```python
from build123d import *

# Parameters (mm, degrees)
SKETCH1_W           = 236
SKETCH1_H           = 236
BOSS_EXTRUDE1_DEPTH = 240
SHELL1_T            = -40
FILLET1_R           = 23
FILLET2_R           = 30
SKETCH3_W           = 80
SKETCH3_H           = 120
CUT_EXTRUDE2_DEPTH  = 240


with BuildPart() as part:
    # Sketch1 → Boss-Extrude1 (new body)
    with BuildSketch(Plane(origin=(0, 0, 0), x_dir=(1, 0, 0), z_dir=(0, 1, 0))):
        with Locations((2.531496063, -48.329724409)):
            Rectangle(SKETCH1_W, SKETCH1_H)
    extrude(amount=BOSS_EXTRUDE1_DEPTH)

    # Shell1
    shell1_openings = [part.faces().sort_by_distance(p)[0] for p in [
        (2.531496063, 240, 48.329724409),
    ]]
    offset(amount=SHELL1_T, openings=shell1_openings, kind=Kind.INTERSECTION)

    # Fillet1
    fillet1_edges = [part.edges().sort_by_distance(p)[0] for p in [
        (-75.468503937, 40, 48.329724409),
        (-75.468503937, 140, -29.670275591),
        (2.531496063, 40, 126.329724409),
        (-75.468503937, 140, 126.329724409),
        (80.531496063, 40, 48.329724409),
        (80.531496063, 140, 126.329724409),
        (2.531496063, 40, -29.670275591),
        (80.531496063, 140, -29.670275591),
    ]]
    fillet(fillet1_edges, radius=FILLET1_R)

    # Fillet2
    fillet2_edges = [part.edges().sort_by_distance(p)[0] for p in [
        (2.531496063, 0, -69.670275591),
        (120.531496063, 0, 48.329724409),
        (2.531496063, 0, 166.329724409),
        (-115.468503937, 0, 48.329724409),
        (-115.468503937, 120, -69.670275591),
        (120.531496063, 120, -69.670275591),
        (120.531496063, 120, 166.329724409),
        (-115.468503937, 120, 166.329724409),
    ]]
    fillet(fillet2_edges, radius=FILLET2_R)

    # Sketch3 → Cut-Extrude2 (cut)
    with BuildSketch(Plane(origin=(120.531496063, 0, 0), x_dir=(0, 0, -1), z_dir=(1, 0, 0))):
        with Locations((-48.329724409, 123)):
            Rectangle(SKETCH3_W, SKETCH3_H)
    extrude(amount=-CUT_EXTRUDE2_DEPTH, mode=Mode.SUBTRACT)


solid = part.part
```
CAD build for the part. Positions are in the model's coordinates, mm. A direction names the side the tool comes from. Round coordinates to 2 decimals unless told otherwise and drop trailing zeros. Loops run counter-clockwise (first coordinate to the right, second up) from the corner with the lowest first, then second, coordinate; pieces in that order, holes last. Notation, with made-up numbers: M 57.5,-27 L 112.5,-27 A26 cw 112.5,-4 Z; hole C -27.75,10 d10. An arc over 180 degrees is marked long. Use a Markdown table: item, result. Add a question column.
(1) Cut at D-D (x = -101). Give the cut face in (y, z), and give its area (3 significant figures).
(2) Cut at C-C (y = 70.5). Give the cut face in (x, z), and give its area (3 significant figures).
(3) Cut at B-B (z = 32.5). Give the cut face in (x, y).
(4) Pull direction Y, two halves, no side cores. Call faces 4 (the face through (-95, 63, 49)), 5 (the face through (73.615, 152.739, 119.771)), 6 (the face through (1, 240, -32)): +Y half, -Y half, draft (parallel to the pull), parting line (faces both ways), or undercut.
(5) Which spindle directions (+Z, -Z, +X, -X, +Y, -Y) get a long thin tool onto all of the face, cutting with end or side? Do faces 1 (the face through (120.531, 134, 89)), 2 (the face through (-75.469, 190, 49)), 3 (the face through (-95, 122, 8.33)). Say none if no direction does.
(6) Drill centre lines: line 1 (X direction, y = 102.5, z = 2.5); line 2 (Y direction, x = 86, z = 43.5); line 3 (Z direction, x = 91.5, y = 100.5). Where is each one in solid material? Low to high.
(7) Cut at A-A (y = 212.5). Give the cut face in (x, z).
Geometry says:
| question | item | result |
|---|---|---|
| 1 | outline | M 4.33,-39.67 A25.67 ccw 30,-65.34 L 240,-65.34 L 240,162 L 30,162 A25.67 ccw 4.33,136.33 Z; hole M 63,8.33 L 183,8.33 L 183,88.33 L 63,88.33 Z |
| 1 | area | 43,700 mm² |
| 2 | outline | M -115.47,-39.67 A30 ccw -85.47,-69.67 L 90.53,-69.67 A30 ccw 120.53,-39.67 L 120.53,8.33 L 80.53,8.33 L 80.53,-6.67 A23 cw 57.53,-29.67 L -52.47,-29.67 A23 cw -75.47,-6.67 L -75.47,8.33 L -115.47,8.33 Z; M -115.47,88.33 L -75.47,88.33 L -75.47,103.33 A23 cw -52.47,126.33 L 57.53,126.33 A23 cw 80.53,103.33 L 80.53,88.33 L 120.53,88.33 L 120.53,136.33 A30 ccw 90.53,166.33 L -85.47,166.33 A30 ccw -115.47,136.33 Z |
| 2 | area | 24,600 mm² |
| 3 | outline | M -115.47,30 A30 ccw -85.47,0 L 90.53,0 A30 ccw 120.53,30 L 120.53,63 L 80.53,63 A23 cw 57.53,40 L -52.47,40 A23 cw -75.47,63 L -115.47,63 Z; M -115.47,183 L -75.47,183 L -75.47,240 L -115.47,240 Z; M 80.53,183 L 120.53,183 L 120.53,240 L 80.53,240 Z |
| 4 | face 4 | undercut |
| 4 | face 5 | draft |
| 4 | face 6 | +Y half |
| 5 | face 1 | +Z, -Z, +X, +Y, -Y |
| 5 | face 2 | +Y |
| 5 | face 3 | +X, -X |
| 6 | line 1 | x = -115.47 to -75.47, 80.53 to 120.53 |
| 6 | line 2 | y = 0 to 63, 183 to 240 |
| 6 | line 3 | z = -69.65 to 8.33, 88.33 to 166.31 |
| 7 | outline | M -115.47,-39.67 A30 ccw -85.47,-69.67 L 90.53,-69.67 A30 ccw 120.53,-39.67 L 120.53,136.33 A30 ccw 90.53,166.33 L -85.47,166.33 A30 ccw -115.47,136.33 Z; hole M -75.47,-6.67 A23 ccw -52.47,-29.67 L 57.53,-29.67 A23 ccw 80.53,-6.67 L 80.53,103.33 A23 ccw 57.53,126.33 L -52.47,126.33 A23 ccw -75.47,103.33 Z |
